```python
from build123d import *

# Parameters (mm, degrees)
F0_W     = 101.6
F0_H     = 76.2
F1_DEPTH = 152.4
F2_W     = 76.2
F2_H     = 25.4
F3_DEPTH = 50.8
F4_R     = 5.08


with BuildPart() as f1:
    # F0 (on Top) → F1 (new body)
    with BuildSketch(Plane.XY):
        with Locations((0.713926, -12.174402)):
            Rectangle(F0_W, F0_H)
    extrude(amount=F1_DEPTH)

    # F2 (on face) → F3 (cut)
    with BuildSketch(Plane.XZ.offset(50.274402)):
        with Locations((0.713926, 129.54)):
            Rectangle(F2_W, F2_H)
        with Locations((0.762346, 93.980033)):
            Rectangle(F2_W, F2_H)
        with Locations((0.810766, 58.420066)):
            Rectangle(F2_W, F2_H)
        with Locations((0.859186, 22.860099)):
            Rectangle(F2_W, F2_H)
    extrude(amount=-F3_DEPTH, mode=Mode.SUBTRACT)

    # F4
    f4_edges = [f1.edges().sort_by_distance(p)[0] for p in [
        (-50.086074, -12.174402, 152.4),
        (51.513926, -12.174402, 152.4),
        (0.713926, 25.925598, 152.4),
        (0.713926, -50.274402, 152.4),
        (51.513926, -50.274402, 76.2),
        (-50.086074, -50.274402, 76.2),
        (-50.086074, 25.925598, 76.2),
        (0.713926, -50.274402, 0),
        (51.513926, -12.174402, 0),
        (0.713926, 25.925598, 0),
        (-50.086074, -12.174402, 0),
    ]]
    fillet(f4_edges, radius=F4_R)


solid = f1.part
```
Check sheet for the modelled part. Datum: model origin and axes. Units: mm. A direction names the side the tool comes from. Give positions to 0.01 mm unless a question says otherwise; leave off trailing zeros. Order: outer loops, then holes, each group sorted by start corner. A loop starts at its lowest first (then second) coordinate and runs counter-clockwise, first axis right, second up. Notation, with made-up numbers: M 84,-7.5 L 140,-7.5 A23 cw 140,25.5 Z; hole C 17.25,60.25 d5. An arc over 180 degrees is marked long. Answer in a Markdown table with one row per item. Add a question column.
Q1. Gauge pin test, flat end, axial feed: pin 1 Ø7.5 at (x, z) = (-7.5, 128) entering from -Y. Record the tip position at first contact, or that the pin passes through.
Q2. Release check for a two-part mould opening along X. For faces 1 (the flat face through (0, -25, 71.12)), 2 (the cylindrical face through (49.986, -48.826, 77.196)), 3 (the cylindrical face through (-48.637, 24.398, 77.196)) record: released by +X, released by -X, zero draft, split by the parting line, or undercut.
Q3. Access from +Z, -Z, +X, -X, +Y, -Y to the whole of each face (thin tool, end or side, straight path). Record for faces 4 (the flat face through (3, 25.926, 75)), 5 (the flat face through (0, -25, 142.24)).
Q4. Thickness scan on L1, parallel to Z at x = 30.5, y = -36.5; L2, parallel to X at y = -11, z = 61.5; L3, parallel to Z at x = -15, y = -46. Record the ranges inside material, lowest first.
Q5. Sectioned sample at A-A, the plane y = -18.5. Record the boundary of the cut face in (x, z), and give its area (3 significant figures).
Q6. Sectioned sample at B-B, the plane x = 36. Record the boundary of the cut face in (y, z).
Q7. Sectioned sample at C-C, the plane z = 95.5. Record the boundary of the cut face in (x, y), and give its area (3 significant figures).
Verdict:
| question | item | result |
|---|---|---|
| 1 | pin 1 | y = 0.53 |
| 2 | face 1 | undercut |
| 2 | face 2 | released by +X |
| 2 | face 3 | released by -X |
| 3 | face 4 | +Z, -Z, +X, -X, +Y |
| 3 | face 5 | -Y |
| 4 | L1 | 0 to 10.16, 35.56 to 45.72, 71.12 to 81.28, 106.68 to 116.84, 142.24 to 152.4 |
| 4 | L2 | -50.09 to -37.29, 38.91 to 51.51 |
| 4 | L3 | 0.06 to 10.16, 35.56 to 45.72, 71.12 to 81.28, 106.68 to 116.84, 142.24 to 152.34 |
| 5 | outline | M -50.09,5.08 A5.08 ccw -45.01,0 L 46.43,0 A5.08 ccw 51.51,5.08 L 51.51,147.32 A5.08 ccw 46.43,152.4 L -45.01,152.4 A5.08 ccw -50.09,147.32 Z; hole M -37.39,116.84 L 38.81,116.84 L 38.81,142.24 L -37.39,142.24 Z; hole M -37.34,81.28 L 38.86,81.28 L 38.86,106.68 L -37.34,106.68 Z; hole M -37.29,45.72 L 38.91,45.72 L 38.91,71.12 L -37.29,71.12 Z; hole M -37.24,10.16 L 38.96,10.16 L 38.96,35.56 L -37.24,35.56 Z |
| 5 | area | 7,720 mm² |
| 6 | outline | M -50.27,5.08 A5.08 ccw -45.19,0 L 20.85,0 A5.08 ccw 25.93,5.08 L 25.93,147.32 A5.08 ccw 20.85,152.4 L -45.19,152.4 A5.08 ccw -50.27,147.32 L -50.27,142.24 L 0.53,142.24 L 0.53,116.84 L -50.27,116.84 L -50.27,106.68 L 0.53,106.68 L 0.53,81.28 L -50.27,81.28 L -50.27,71.12 L 0.53,71.12 L 0.53,45.72 L -50.27,45.72 L -50.27,35.56 L 0.53,35.56 L 0.53,10.16 L -50.27,10.16 Z |
| 7 | outline | M -50.09,-45.19 A5.08 ccw -45.01,-50.27 L -37.34,-50.27 L -37.34,0.53 L 38.86,0.53 L 38.86,-50.27 L 46.43,-50.27 A5.08 ccw 51.51,-45.19 L 51.51,25.93 L -45.01,25.93 A5.08 ccw -50.09,20.85 Z |
| 7 | area | 3,850 mm² |
